Print and shaded views of the part. All mm, measured from the part's lowest x, y and z. A direction names the side the tool comes from. Give positions to 0.01 mm unless a question says otherwise; leave off trailing zeros. Loops run counter-clockwise (first coordinate to the right, second up) from the corner with the lowest first, then second, coordinate; pieces in that order, holes last.
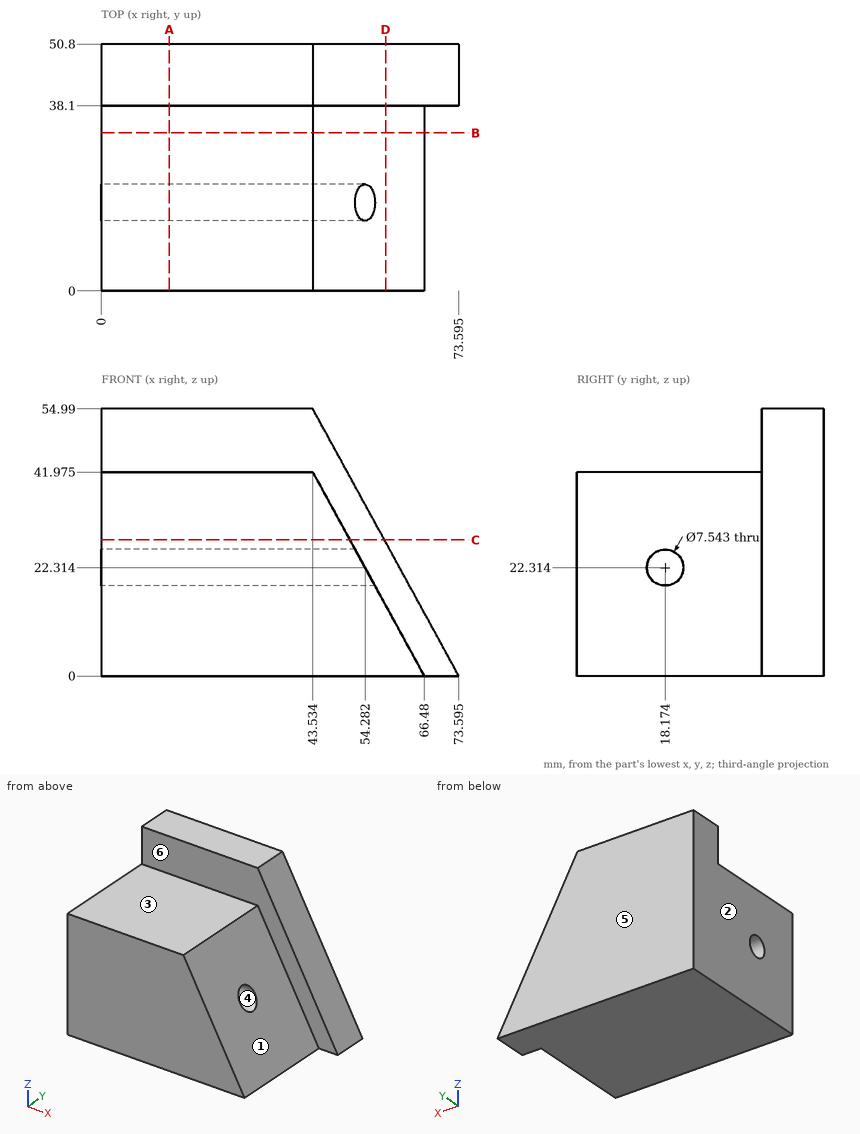
1. Drop flat-ended pins along their axis: pin 1 (11.5 mm diameter, centred on x = 19, y = 11, fed in from +Z) (1 decimal); pin 2 (6 mm diameter, centred on y = 15, z = 30, fed in from +X); pin 3 (4 mm diameter, centred on x = 33.5, z = 45.5, fed in from -Y). Give the stop position or say it passes through.
Responses:
pin 1: stops at z = 42
pin 2: stops at x = 51.72
pin 3: stops at y = 38.1
2. Saw through at B-B, the plane y = 32.5. List the corners of the cut face in (x, z) (1 decimal), and give its area (3 significant figures).
Responses:
outline: (0, 0) - (66.5, 0) - (43.5, 42) - (0, 42) - close
area: 2,310 mm2
3. Saw through at A-A, the plane x = 14. List the corners of the cut face in (y, z) (1 decimal), and give its area (3 significant figures).
Responses:
outline: (0, 0) - (50.8, 0) - (50.8, 55) - (38.1, 55) - (38.1, 42) - (0, 42) - close; hole circle Ø7.5 at (18.2, 22.3)
area: 2,250 mm2
4. Saw through at C-C, the plane z = 28. List the corners of the cut face in (x, y).
Responses:
outline: (0, 0) - (51.17, 0) - (51.17, 38.1) - (58.29, 38.1) - (58.29, 50.8) - (0, 50.8) - close
5. Tool access for the marked faces 1 and 2: list every direction of +Z, -Z, +X, -X, +Y, -Y with a clear straight run to the whole face (end or side of a thin tool).
Responses:
face 1: +Z, +X, -Y
face 2: +Z, -Z, -X, +Y, -Y
6. Probe line 1 along Z through (x, y) = (11, 9) (1 decimal); line 2 along Z through (x, y) = (6, 19.5) (1 decimal); line 3 along Z through (x, y) = (15, 16.5) (1 decimal). List the from-to ranges inside material, lowest first.
Responses:
line 1: z = 0 to 42
line 2: z = 0 to 18.8, 25.8 to 42
line 3: z = 0 to 18.9, 25.7 to 42
7. Pull direction Y, two halves, no side cores. Call the marked faces 3, 4, 5 and 6: released by +Y, released by -Y, zero draft, split by the parting line, or undercut.
Responses:
face 3: zero draft
face 4: undercut
face 5: released by +Y
face 6: released by -Y
8. Saw through at D-D, the plane x = 58.5. List the corners of the cut face in (y, z), and give its area (3 significant figures).
Responses:
outline: (0, 0) - (50.8, 0) - (50.8, 27.61) - (38.1, 27.61) - (38.1, 14.6) - (0, 14.6) - close
area: 907 mm2
